from build123d import *

# Parameters (mm, degrees)
BOSS_EXTRUDE1_DEPTH   = 327.5
BOSS_EXTRUDE1_2_DEPTH = 327.5
BOSS_EXTRUDE2_DEPTH   = 2
BOSS_EXTRUDE4_DEPTH   = 1
SKETCH4_W             = 100
SKETCH4_H             = 8.5
BOSS_EXTRUDE5_DEPTH   = 2
BOSS_EXTRUDE6_DEPTH   = 1
SKETCH7_R             = 5
SKETCH7_W             = 96
SKETCH7_H             = 1
CUT_EXTRUDE2_DEPTH    = 1
SKETCH8_W             = 100
SKETCH8_H             = 13.5
CUT_EXTRUDE3_DEPTH    = 400
SKETCH9_W             = 1
SKETCH9_H             = 5
CUT_EXTRUDE4_DEPTH    = 84.5
BOSS_EXTRUDE8_DEPTH   = 1
SKETCH15_W            = 110.261376908
SKETCH15_H            = 36.265100391
CUT_EXTRUDE7_DEPTH    = 400


with BuildPart() as part:
    # Sketch1 → Boss-Extrude1 (new body)
    with BuildSketch(Plane.XY):
        Polygon((0, 0), (0, 8.5), (1, 8.5), (1, 13.5), (2, 13.5), (2, 2), (13.5, 2), (13.5, 1), (8.5, 1), (8.5, 0), align=None)
    extrude(amount=BOSS_EXTRUDE1_DEPTH)



with BuildPart() as body_2:
    # Sketch1 → Boss-Extrude1 2 (new body)
    with BuildSketch(Plane.XY):
        Polygon((100, 0), (91.5, 0), (91.5, 1), (86.5, 1), (86.5, 2), (98, 2), (98, 13.5), (99, 13.5), (99, 8.5), (100, 8.5), align=None)
    extrude(amount=BOSS_EXTRUDE1_2_DEPTH)


with BuildPart() as part_1:
    add(part.part)

    add(body_2.part)  # Boss-Extrude2 merges body 2
    # Sketch2 → Boss-Extrude2 (add)
    with BuildSketch(Plane(origin=(0, 2, 0), x_dir=(1, 0, 0), z_dir=(0, 1, 0))):
        Polygon((86.5, 0), (13.5, -73), (13.5, -85.02081528), (86.5, -12.02081528), align=None)
    extrude(amount=-BOSS_EXTRUDE2_DEPTH)

    # Sketch3 → Boss-Extrude4 (add)
    with BuildSketch(Plane.XZ.offset(-1)):
        Polygon((13.5, 73), (13.5, 85.02081528), (8.5, 90.02081528), (8.5, 78), align=None)
        Polygon((86.5, 0), (86.5, 12.02081528), (91.5, 7.02081528), (91.5, 0), align=None)
    extrude(amount=BOSS_EXTRUDE4_DEPTH)

    # Sketch4 → Boss-Extrude5 (add)
    with BuildSketch(Plane.XZ):
        with Locations((50, 323.25)):
            Rectangle(SKETCH4_W, SKETCH4_H)
    extrude(amount=-BOSS_EXTRUDE5_DEPTH)

    # Sketch7 → Cut-Extrude2 (cut)
    with BuildSketch(Plane(origin=(0, 2, 0), x_dir=(1, 0, 0), z_dir=(0, 1, 0))):
        with Locations((26.5, -326.5)):
            Circle(SKETCH7_R)
        with Locations((73.5, -326.5)):
            Circle(SKETCH7_R)
        with Locations((50, -327)):
            Rectangle(SKETCH7_W, SKETCH7_H)
    extrude(amount=-CUT_EXTRUDE2_DEPTH, mode=Mode.SUBTRACT)


with BuildPart() as body_2_2:
    # Sketch5 → Boss-Extrude6 (new body)
    with BuildSketch(Plane(origin=(0, 2, 0), x_dir=(1, 0, 0), z_dir=(0, 1, 0))):
        Polygon((13.5, -65.928932188), (79.428932188, 0), (86.5, 0), (13.5, -73), align=None)
    extrude(amount=-BOSS_EXTRUDE6_DEPTH)


with BuildPart() as body_3:
    # Mirror1: mirrored copy
    add(body_2_2.part.mirror(Plane(origin=(1, 13.5, 327.5), x_dir=(0, 0, 1), z_dir=(0, -1, 0))))


with BuildPart() as body_4:
    # Mirror1 2: mirrored copy
    add(part_1.part.mirror(Plane(origin=(1, 13.5, 327.5), x_dir=(0, 0, 1), z_dir=(0, -1, 0))))

    # Sketch9 → Cut-Extrude4 (cut)
    with BuildSketch(Plane(origin=(0, 0, 0), x_dir=(-1, 0, 0), z_dir=(0, 0, -1))):
        with Locations((-1.5, 16)):
            Rectangle(SKETCH9_W, SKETCH9_H)
    extrude(amount=-CUT_EXTRUDE4_DEPTH, mode=Mode.SUBTRACT)


with BuildPart() as cut_extrude3_tool:
    # Sketch8 → Cut-Extrude3 (new body)
    with BuildSketch(Plane(origin=(0, 0, 0), x_dir=(-1, 0, 0), z_dir=(0, 0, -1))):
        with Locations((-50, 6.75)):
            Rectangle(SKETCH8_W, SKETCH8_H)
    extrude(amount=-CUT_EXTRUDE3_DEPTH)


with BuildPart() as part_2:
    add(part_1.part)

    # Cut-Extrude3: cut by cut_extrude3_tool
    add(cut_extrude3_tool.part, mode=Mode.SUBTRACT)


with BuildPart() as body_2_2_1:
    add(body_2_2.part)

    # Cut-Extrude3: cut by cut_extrude3_tool
    add(cut_extrude3_tool.part, mode=Mode.SUBTRACT)


with BuildPart() as body_3_2:
    # Sketch14 → Boss-Extrude8 (new body)
    with BuildSketch(Plane(origin=(0, 27, 0), x_dir=(1, 0, 0), z_dir=(0, 1, 0))):
        Polygon((8.5, 0), (8.5, -78), (86.5, 0), align=None)
    extrude(amount=BOSS_EXTRUDE8_DEPTH)


with BuildPart() as cut_extrude7_tool:
    # Sketch15 → Cut-Extrude7 (new body)
    with BuildSketch(Plane(origin=(0, 0, 0), x_dir=(-1, 0, 0), z_dir=(0, 0, -1))):
        with Locations((-44.869311546, 8.867449804)):
            Rectangle(SKETCH15_W, SKETCH15_H)
    extrude(amount=-CUT_EXTRUDE7_DEPTH)


with BuildPart() as body_3_1:
    add(body_3.part)

    # Cut-Extrude7: cut by cut_extrude7_tool
    add(cut_extrude7_tool.part, mode=Mode.SUBTRACT)


with BuildPart() as body_4_1:
    add(body_4.part)

    # Cut-Extrude7: cut by cut_extrude7_tool
    add(cut_extrude7_tool.part, mode=Mode.SUBTRACT)


solid = body_3_2.part
Check sheet for the modelled part. Datum: model origin and axes. Units: mm. Round coordinates to 2 decimals unless told otherwise and drop trailing zeros. Order: outer loops, then holes, each group sorted by start corner. A loop starts at its lowest first (then second) coordinate and runs counter-clockwise, first axis right, second up.
(1) Scan lines: probe 1 along X at (y, z) = (27.15, 12.5); probe 2 along Z at (x, y) = (68.5, 27.5); probe 3 along X at (y, z) = (27.35, 47). Record each from-to range of solid material in increasing order.
(2) Cross-section at B-B, the plane x = 70. Enter the section's corners in (y, z), and give its area (3 significant figures).
(3) Cross-section at A-A, the plane z = 68. Enter the section's corners in (x, y).
(4) Cross-section at C-C, the plane y = 27.35. Enter the section's corners in (x, z), and give its area (3 significant figures).
Check sheet entries:
1. probe 1: x = 8.5 to 74
1. probe 2: z = 0 to 18
1. probe 3: x = 8.5 to 39.5
2. outline: (27, 0) - (28, 0) - (28, 16.5) - (27, 16.5) - close
2. area: 16.5 mm2
3. outline: (8.5, 27) - (18.5, 27) - (18.5, 28) - (8.5, 28) - close
4. outline: (8.5, 0) - (86.5, 0) - (8.5, 78) - close
4. area: 3,040 mm2
